from build123d import *

# Parameters (mm, degrees)
SKETCH1_R           = 26.83
SKETCH1_R_2         = 7
SKETCH1_R_3         = 2
BOSS_EXTRUDE1_DEPTH = 2.5
CUT_EXTRUDE1_DEPTH  = 10
CUT_EXTRUDE2_DEPTH  = 10


with BuildPart() as part:
    # Sketch1 → Boss-Extrude1 (new body)
    with BuildSketch(Plane(origin=(0, 0, 0), x_dir=(1, 0, 0), z_dir=(0, 1, 0))):
        Circle(SKETCH1_R)
        Circle(SKETCH1_R_2, mode=Mode.SUBTRACT)
        with Locations((-16.000000001, 16.000000001)):
            Circle(SKETCH1_R_3, mode=Mode.SUBTRACT)
        with Locations((16.000000001, 16.000000001)):
            Circle(SKETCH1_R_3, mode=Mode.SUBTRACT)
        with Locations((16.000000001, -16.000000001)):
            Circle(SKETCH1_R_3, mode=Mode.SUBTRACT)
        with Locations((-16.000000001, -16.000000001)):
            Circle(SKETCH1_R_3, mode=Mode.SUBTRACT)
    extrude(amount=BOSS_EXTRUDE1_DEPTH)

    # Sketch2 → Cut-Extrude1 (cut)
    with BuildSketch(Plane(origin=(0, 2.5, 0), x_dir=(1, 0, 0), z_dir=(0, 1, 0))):
        with BuildLine():
            ThreePointArc((-6.000000001, 8.000000001), (-9.414213563, 9.414213563), (-8.000000001, 6.000000001))
            Line((-8.000000001, 6.000000001), (-8.000000001, 8.000000001))
            Line((-8.000000001, 8.000000001), (-6.000000001, 8.000000001))
        make_face()
        with BuildLine():
            Line((-8.000000001, 8.000000001), (-8.000000001, 6.000000001))
            ThreePointArc((-8.000000001, 6.000000001), (-6.585786438, 6.585786438), (-6.000000001, 8.000000001))
            Line((-6.000000001, 8.000000001), (-8.000000001, 8.000000001))
        make_face()
        with BuildLine():
            ThreePointArc((6.000000001, 8.000000001), (6.585786438, 6.585786438), (8.000000001, 6.000000001))
            Line((8.000000001, 6.000000001), (8.000000001, 8.000000001))
            Line((8.000000001, 8.000000001), (6.000000001, 8.000000001))
        make_face()
        with BuildLine():
            Line((8.000000001, 8.000000001), (8.000000001, 6.000000001))
            ThreePointArc((8.000000001, 6.000000001), (9.414213563, 6.585786438), (10.000000001, 8.000000001))
            ThreePointArc((10.000000001, 8.000000001), (8.000000001, 10.000000001), (6.000000001, 8.000000001))
            Line((6.000000001, 8.000000001), (8.000000001, 8.000000001))
        make_face()
        with BuildLine():
            Line((-6.000000001, -8.000000001), (-8.000000001, -8.000000001))
            Line((-8.000000001, -8.000000001), (-8.000000001, -6.000000001))
            ThreePointArc((-8.000000001, -6.000000001), (-9.414213563, -9.414213563), (-6.000000001, -8.000000001))
        make_face()
        with BuildLine():
            ThreePointArc((-6.000000001, -8.000000001), (-6.152240936, -7.234633136), (-6.585786438, -6.585786438))
            Line((-6.585786438, -6.585786438), (-8.000000001, -8.000000001))
            Line((-8.000000001, -8.000000001), (-6.000000001, -8.000000001))
        make_face()
        with BuildLine():
            Line((-8.000000001, -8.000000001), (-6.585786438, -6.585786438))
            ThreePointArc((-6.585786438, -6.585786438), (-7.234633136, -6.152240936), (-8.000000001, -6.000000001))
            Line((-8.000000001, -6.000000001), (-8.000000001, -8.000000001))
        make_face()
        with BuildLine():
            ThreePointArc((8.000000001, -6.000000001), (6.585786438, -6.585786438), (6.000000001, -8.000000001))
            Line((6.000000001, -8.000000001), (8.000000001, -8.000000001))
            Line((8.000000001, -8.000000001), (8.000000001, -6.000000001))
        make_face()
        with BuildLine():
            Line((8.000000001, -8.000000001), (6.000000001, -8.000000001))
            ThreePointArc((6.000000001, -8.000000001), (8.000000001, -10.000000001), (10.000000001, -8.000000001))
            ThreePointArc((10.000000001, -8.000000001), (9.414213563, -6.585786438), (8.000000001, -6.000000001))
            Line((8.000000001, -6.000000001), (8.000000001, -8.000000001))
        make_face()
    extrude(amount=-CUT_EXTRUDE1_DEPTH, mode=Mode.SUBTRACT)

    # Sketch3 → Cut-Extrude2 (cut)
    with BuildSketch(Plane(origin=(0, 2.5, 0), x_dir=(1, 0, 0), z_dir=(0, 1, 0))):
        with BuildLine():
            Line((-19.833935995, -18.068311569), (-19.833935995, 18.068311569))
            ThreePointArc((-19.833935995, 18.068311569), (-26.83, 0), (-19.833935995, -18.068311569))
        make_face()
        with BuildLine():
            Line((-18.068311569, 19.833935995), (18.068311569, 19.833935995))
            ThreePointArc((18.068311569, 19.833935995), (0, 26.83), (-18.068311569, 19.833935995))
        make_face()
        with BuildLine():
            ThreePointArc((26.83, 0), (25.019926086, 9.687734443), (19.833935995, 18.068311569))
            Line((19.833935995, 18.068311569), (19.833935995, -18.068311569))
            ThreePointArc((19.833935995, -18.068311569), (25.019926086, -9.687734443), (26.83, 0))
        make_face()
        with BuildLine():
            ThreePointArc((-18.068311569, -19.833935995), (0, -26.83), (18.068311569, -19.833935995))
            Line((18.068311569, -19.833935995), (-18.068311569, -19.833935995))
        make_face()
    extrude(amount=-CUT_EXTRUDE2_DEPTH, mode=Mode.SUBTRACT)


solid = part.part
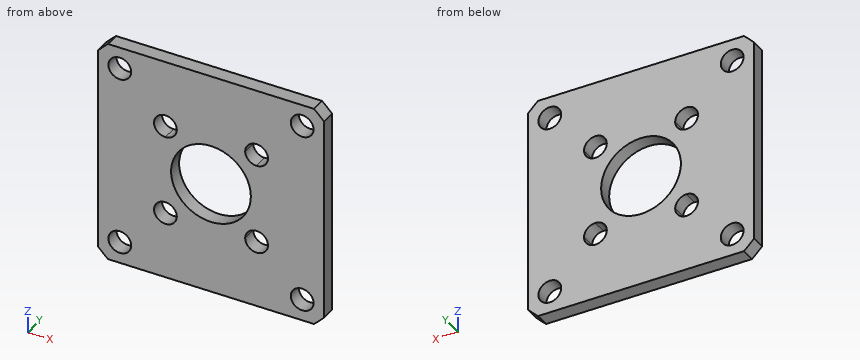
Could you check a few things on this model? Use its own coordinates, in mm. Give positions to 0.01 mm unless a question says otherwise; leave off trailing zeros. Write each loop counter-clockwise with the first axis right and the second up, starting at its lowest first coordinate (ties: lowest second). Pieces come first, ordered by that corner, then holes. Notation, with made-up numbers: (-16, 51) -> (3, 51) arc R22 cw to (3, 61) -> close; hole circle Ø6 at (-12, -5.5). An arc over 180 degrees is marked (long way). Answer as CSV lines item,"result". Start each with the question number.
(1) If we section it at D-D, the plane y = 1.5: Give the number of separate pieces and of enclosed holes in the cut face, and give its area (3 significant figures).
(2) If we section it at C-C, the plane x = 0: Write out the boundary of the cut face in (y, z), and give its area (3 significant figures).
(3) Please list where these lines run through material, in increasing order: line 1 (Z direction, x = -8, y = 0.5); line 2 (Z direction, x = 14.5, y = 1.1); line 3 (X direction, y = 2.25, z = 16.5).
(4) If we section it at A-A, the plane x = 16: Write out the boundary of the cut face in (y, z).
(5) If we section it at B-B, the plane z = 0: Write out the boundary of the cut face in (x, y), and give its area (3 significant figures).
Answer list:
1,separate pieces,"1"
1,enclosed holes,"9"
1,area,"1,310 mm^2"
2,outline,"(0, -19.83) -> (2.5, -19.83) -> (2.5, -7) -> (0, -7) -> close; (0, 7) -> (2.5, 7) -> (2.5, 19.83) -> (0, 19.83) -> close"
2,area,"64.2 mm^2"
3,line 1,"-19.83 to -10, -6 to 6, 10 to 19.83"
3,line 2,"-19.83 to -17.32, -14.68 to 14.68, 17.32 to 19.83"
3,line 3,"-19.83 to -17.94, -14.06 to 14.06, 17.94 to 19.83"
4,outline,"(0, -19.83) -> (2.5, -19.83) -> (2.5, -18) -> (0, -18) -> close; (0, -14) -> (2.5, -14) -> (2.5, 14) -> (0, 14) -> close; (0, 18) -> (2.5, 18) -> (2.5, 19.83) -> (0, 19.83) -> close"
5,outline,"(-19.83, 0) -> (-7, 0) -> (-7, 2.5) -> (-19.83, 2.5) -> close; (7, 0) -> (19.83, 0) -> (19.83, 2.5) -> (7, 2.5) -> close"
5,area,"64.2 mm^2"
